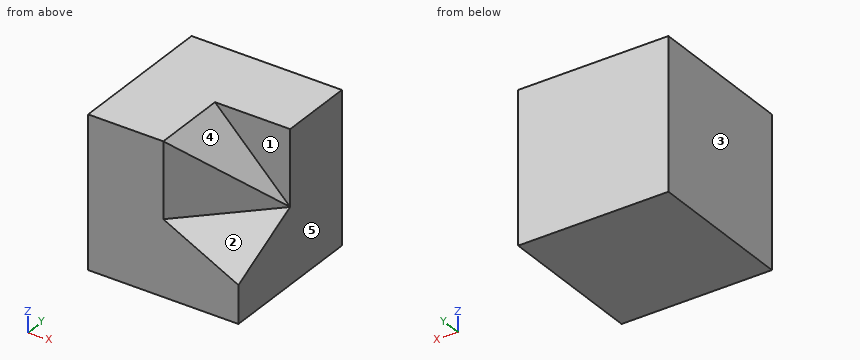
```python
from build123d import *

# Parameters (mm, degrees)
F0_W      = 40
F0_H      = 40
F1_DEPTH  = 40
F2_W      = 20
F2_H      = 20
F3_DEPTH  = 20
F7_DEPTH  = 24.4958974278
F9_DEPTH  = 20
F11_DEPTH = 20


with BuildPart() as f1:
    # F0 (on Front) → F1 (new body)
    with BuildSketch(Plane.XZ):
        with Locations((20, 20)):
            Rectangle(F0_W, F0_H)
    extrude(amount=F1_DEPTH)

    # F2 (on face) → F3 (cut)
    with BuildSketch(Plane.XZ.offset(40)):
        with Locations((30, 30)):
            Rectangle(F2_W, F2_H)
    extrude(amount=-F3_DEPTH, mode=Mode.SUBTRACT)

    # F6 (on 3pt) → F7 (cut, through all)
    with BuildSketch(Plane(origin=(16.6666666667, -16.6666666667, 33.3333333333), x_dir=(0.9128709292, 0.1825741858, -0.3651483717), z_dir=(-0.4082482905, 0.4082482905, -0.8164965809))):
        Polygon((3.6514837167, 26.83281573), (25.5603860169, 8.94427191), (25.5603860169, 31.304951685), align=None)
    extrude(amount=-F7_DEPTH, mode=Mode.SUBTRACT)

    # F8 (on face) → F9 (join, through all)
    with BuildSketch(Plane.XZ.offset(20)):
        Polygon((40, 20), (20, 40), (20, 20), align=None)
    extrude(amount=F9_DEPTH)

    # F10 (on face) → F11 (cut, through all)
    with BuildSketch(Plane(origin=(0, 0, 20), x_dir=(1, 0, 0), z_dir=(0, 0, -1))):
        Polygon((20, 40), (40, 20), (40, 40), align=None)
    extrude(amount=-F11_DEPTH, mode=Mode.SUBTRACT)


solid = f1.part
```
Geometry: final body of the model. Coordinates: model frame, mm. Face numbers are marked on the shaded views. A direction names the side the tool comes from. Coordinates: 2 decimals unless noted, no trailing zeros. Order: outer loops, then holes, each group sorted by start corner. A loop starts at its lowest first (then second) coordinate and runs counter-clockwise, first axis right, second up. Notation, with made-up numbers: (74, 50) - (113, 50) arc R34 ccw to (113, 85) - close; hole circle Ø8 at (0.5, -10). An arc over 180 degrees is marked (long way). Return JSON: item names as keys, results as strings. Group by question number.
1. Cut plane B-B (z = 30.5). Output: boundary loops of the cut face in (x, y).
2. Pin query (flat end, axial travel): pin 1 (5 mm diameter, centred on x = 27.5, y = -23.5, fed in from +Z). Return the tip coordinate at first contact, or that it passes through.
3. Material intervals for line 1 along X through (y, z) = (-36, 14.5); line 2 along Z through (x, y) = (24, -31); line 3 along Z through (x, y) = (23, -35.5), sorted ascending. Write a range as [from, to].
4. Cut plane D-D (x = 23.5). Output: boundary loops of the cut face in (y, z).
5. Cut plane C-C (y = -36.5). Output: boundary loops of the cut face in (x, z), plus the area to 3 significant figures.
6. Set-up query: the marked faces 4 and 5. Return all of +Z, -Z, +X, -X, +Y, -Y with unobstructed straight access to the full face (end or side cutting, diameter ignored); none if empty.
7. Pull-direction query (X, two-part tool) for the marked faces 1, 2 and 3; classes: pulls with the +X half, pulls with the -X half, needs draft (parallel to the pull), parting line crosses it, or undercut.
8. Cut plane A-A (x = 37.5). Output: boundary loops of the cut face in (y, z), plus the area to 3 significant figures.
Resolved:
{
 "1": {"outline": "(0, -40) - (20, -40) - (29.5, -30.5) - (29.5, -20) - (40, -20) - (40, 0) - (0, 0) - close"},
 "2": {"pin 1": "stops at z = 35"},
 "3": {"line 1": "x = [0, 35]", "line 2": "z = [0, 36]", "line 3": "z = [0, 37]"},
 "4": {"outline": "(-40, 0) - (0, 0) - (0, 40) - (-20, 40) - (-20, 36.5) - (-36.5, 36.5) - (-36.5, 20) - (-40, 18.25) - close"},
 "5": {"outline": "(0, 0) - (40, 0) - (40, 11.75) - (23.5, 20) - (23.5, 36.5) - (20, 40) - (0, 40) - close", "area": "1,200 mm²"},
 "6": {"face 4": "+Z, +X, -Y", "face 5": "+Z, -Z, +X, +Y, -Y"},
 "7": {"face 1": "needs draft", "face 2": "pulls with the +X half", "face 3": "pulls with the -X half"},
 "8": {"outline": "(-40, 0) - (0, 0) - (0, 40) - (-20, 40) - (-20, 22.5) - (-22.5, 22.5) - (-22.5, 20) - (-40, 11.25) - close", "area": "1,130 mm²"}
}
